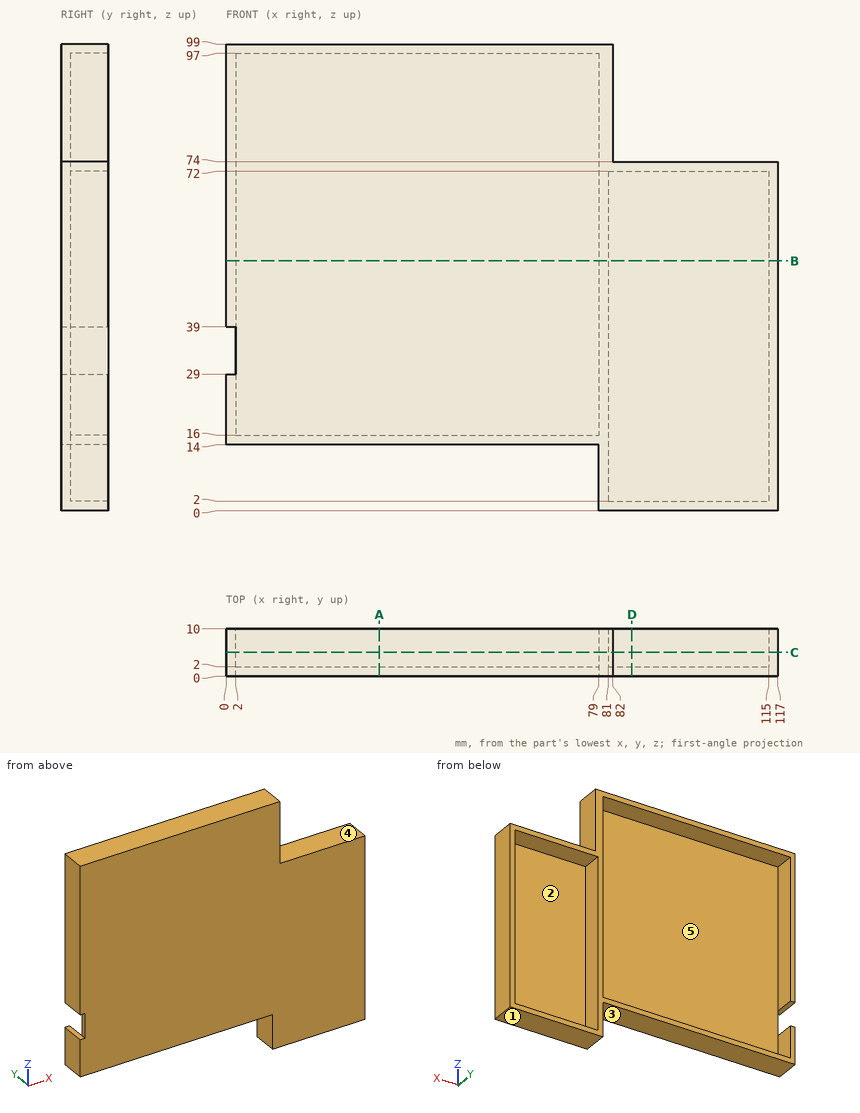
Geometry check sheet. Reference: drawing and pictorial views, mm from the part's lowest x, y, z. A direction names the side the tool comes from. Coordinates: 2 decimals unless noted, no trailing zeros. Write each loop counter-clockwise with the first axis right and the second up, starting at its lowest first coordinate (ties: lowest second). Pieces come first, ordered by that corner, then holes. Notation, with made-up numbers: (89, 54.25) - (115, 54.25) arc R21 ccw to (115, 61.25) - close; hole circle Ø4 at (-4, -34). An arc over 180 degrees is marked (long way). Write item = value, one per line.
Q1. Cross-section at A-A (x = 32.5). Enter the section's corners in (y, z), plus the area to 3 significant figures.
Answer:
outline = (0, 14) - (10, 14) - (10, 16) - (2, 16) - (2, 97) - (10, 97) - (10, 99) - (0, 99) - close
area = 202 mm²
Q2. Material ranges on L1, parallel to X at y = 4.5, z = 42; L2, parallel to Z at x = 110, y = 5.5; L3, parallel to X at y = 4, z = 10, recorded low to high. Write a range as from..to.
Answer:
L1 = 0..2, 79..81, 115..117
L2 = 0..2, 72..74
L3 = 79..81, 115..117
Q3. Cross-section at B-B (z = 53). Enter the section's corners in (x, y), plus the area to 3 significant figures.
Answer:
outline = (0, 0) - (117, 0) - (117, 10) - (115, 10) - (115, 2) - (81, 2) - (81, 10) - (79, 10) - (79, 2) - (2, 2) - (2, 10) - (0, 10) - close
area = 282 mm²
Q4. Cross-section at D-D (x = 86). Enter the section's corners in (y, z).
Answer:
outline = (0, 0) - (10, 0) - (10, 2) - (2, 2) - (2, 72) - (10, 72) - (10, 74) - (0, 74) - close
Q5. Mould release check, pull along X, two halves, no side actions. Record for the marked faces 1 and 2: released by +X, released by -X, zero draft, split by the parting line, or undercut.
Answer:
face_1 = zero draft
face_2 = undercut
Q6. Go/stop test with flat-tipped pins: pin 1 Ø0.6 at (y, z) = (0.5, 31.5) entering from -X; pin 2 Ø12 at (x, z) = (77.5, 75) entering from -Y; pin 3 Ø2.5 at (y, z) = (6.5, 80.5) entering from +X; pin 4 Ø5 at (x, z) = (15, 21) entering from +Y. Record where each tip stops, or that it passes through.
Answer:
pin_1 = 2
pin_2 = 0
pin_3 = 82
pin_4 = 2
Q7. Access from +Z, -Z, +X, -X, +Y, -Y to the whole of each face (thin tool, end or side, straight path). Record for the marked faces 3, 4 and 5.
Answer:
face_3 = -Z, -X, +Y, -Y
face_4 = +Z, +X, +Y, -Y
face_5 = +Y
Q8. Cross-section at C-C (y = 5). Enter the section's corners in (x, z), plus the area to 3 significant figures.
Answer:
outline = (0, 14) - (79, 14) - (79, 0) - (117, 0) - (117, 74) - (82, 74) - (82, 99) - (0, 99) - (0, 39) - (2, 39) - (2, 97) - (79, 97) - (79, 16) - (2, 16) - (2, 29) - (0, 29) - close; hole (81, 2) - (115, 2) - (115, 72) - (81, 72) - close
area = 965 mm²
